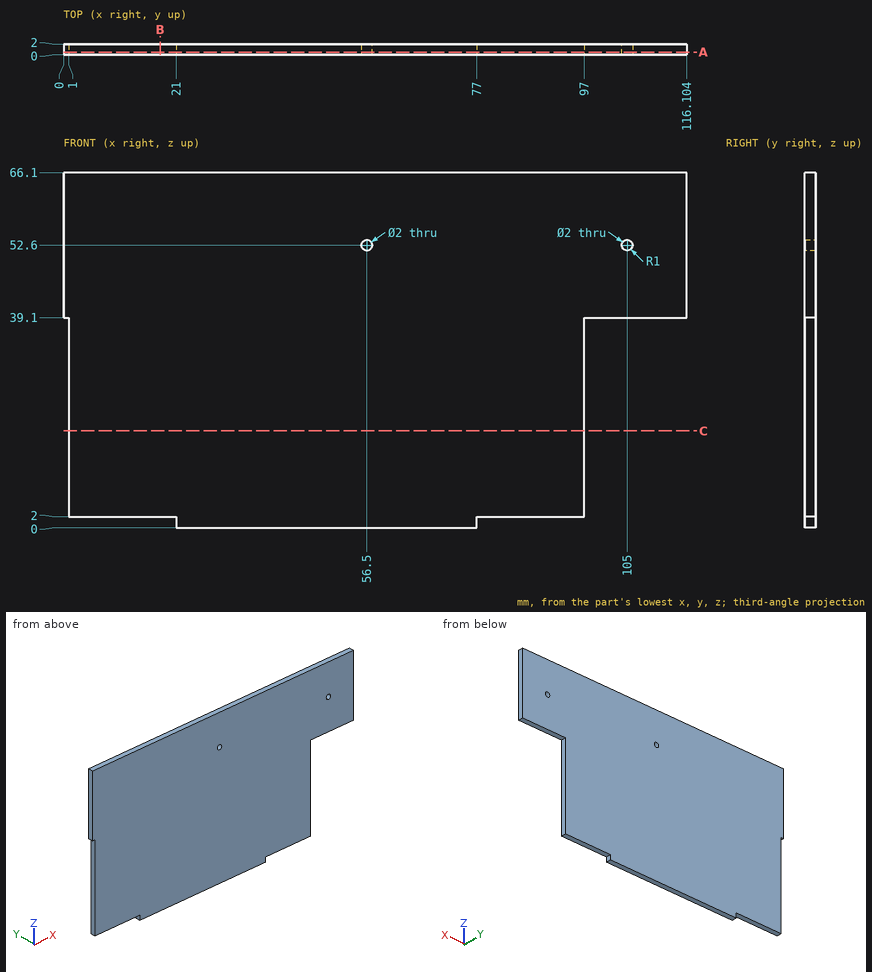
Part print with two shaded views. Sizes in mm from the minimum x, y, z corner. Coordinates: 2 decimals unless noted, no trailing zeros. Order: outer loops, then holes, each group sorted by start corner. A loop starts at its lowest first (then second) coordinate and runs counter-clockwise, first axis right, second up. Notation, with made-up numbers: (68, -7) - (124, -7) arc R13 cw to (124, 5) - close; hole circle Ø3 at (-1, 23). An arc over 180 degrees is marked (long way). Answer in a Markdown table with one row per item.
1. Slice it at C-C, the plane z = 18. List the corners of the cut face in (x, y).
Answer:
| item | result |
|---|---|
| outline | (1, 0) - (97, 0) - (97, 2) - (1, 2) - close |
2. Drill centre lines: L1, parallel to Z at x = 56.5, y = 1; L2, parallel to X at y = 1.1, z = 53; L3, parallel to X at y = 1.5, z = 12. Where is each one in solid material? Low to high. Write a range as from..to.
Answer:
| item | result |
|---|---|
| L1 | 0..51.6, 53.6..66.1 |
| L2 | 0..55.58, 57.42..104.08, 105.92..116.1 |
| L3 | 1..97 |
3. Slice it at A-A, the plane y = 0.5. List the corners of the cut face in (x, z), then the cut area to 3 significant figures.
Answer:
| item | result |
|---|---|
| outline | (0, 39.1) - (1, 39.1) - (1, 2) - (21, 2) - (21, 0) - (77, 0) - (77, 2) - (97, 2) - (97, 39.1) - (116.1, 39.1) - (116.1, 66.1) - (0, 66.1) - close; hole circle Ø2 at (56.5, 52.6); hole circle Ø2 at (105, 52.6) |
| area | 6,800 mm² |
4. Slice it at B-B, the plane x = 18. List the corners of the cut face in (y, z).
Answer:
| item | result |
|---|---|
| outline | (0, 2) - (2, 2) - (2, 66.1) - (0, 66.1) - close |
5. Flat gauge pins, fed straight in: P1, Ø0.8, axis at x = 0.5, y = 1, coming from the -Z side; P2, Ø1.8, axis at x = 56.5, z = 52.6, coming from the +Y side; P3, Ø1, axis at y = 0.5, z = 1, coming from the -X side; P4, Ø0.6, axis at y = 1, z = 28.5, coming from the -X side. Where does each tip first touch, or does it go through?
Answer:
| item | result |
|---|---|
| P1 | z = 39.1 |
| P2 | through |
| P3 | x = 21 |
| P4 | x = 1 |
